The model under review builds one solid part; all positions refer to its coordinate system, in mm. Face numbers are marked on the shaded views. A direction names the side the tool comes from. Coordinates: 2 decimals unless noted, no trailing zeros. Loops run counter-clockwise (first coordinate to the right, second up) from the corner with the lowest first, then second, coordinate; pieces in that order, holes last. Notation, with made-up numbers: (33.25, 49) - (85.25, 49) arc R18 cw to (85.25, 56) - close; hole circle Ø5 at (51, 79). An arc over 180 degrees is marked (long way). Answer in a Markdown table with one row per item. Add a question column.
(1) Mouldability with a two-part tool opening along X and no side actions: class the marked faces 3, 4, 5 and 6 as +X half, -X half, draft (parallel to the pull), parting line (faces both ways), or undercut.
(2) We need section A-A on z = 11.5. Write out the cut boundary in (x, y).
(3) For line 1 along X through (y, z) = (-11.5, 9.75); line 2 along X through (y, z) = (-16, 0.5); line 3 along Z through (x, y) = (2, -21.5), list the stretches that pass through material, from the lowest coordinate up.
(4) We need section D-D on y = -2.5. Write out the cut boundary in (x, z), plus the area to 3 significant figures.
(5) Machinability: for the marked faces 1 and 2, which of the approach directions +Z, -Z, +X, -X, +Y, -Y give a long, thin tool a straight path to every point of the face, cutting with its end or side? Answer none if there is none.
(6) For P1, Ø0.6, axis at x = 0.5, y = -20, coming from the +Z side; P2, Ø2, axis at x = 0, y = -12, coming from the +Z side; P3, Ø1.6, axis at x = -0.5, z = 12.5, coming from the -Y side; P4, Ø2, axis at y = -4, z = -10.5, coming from the +X side, all flat-tipped, find the tip position at first contact; note any pin that passes through.
(7) We need section C-C on y = -23. Write out the cut boundary in (x, z), plus the area to 3 significant figures.
from build123d import *

# Parameters (mm, degrees)
F0_W     = 14
F0_H     = 5
F1_DEPTH = 2
F2_W     = 13
F2_H     = 5
F3_DEPTH = 31
F4_W     = 2
F4_H     = 1.2
F5_DEPTH = 2


with BuildPart() as f1:
    # F0 (on Front) → F1 (new body)
    with BuildSketch(Plane.XZ):
        Polygon((2.468578, 14), (-2.468578, 14), (-7.107986, 12.311393), (-10.890067, 9.137851), (-13.358645, 4.862149), (-14.215973, 0), (-13.358645, -4.862149), (-10.890067, -9.137851), (-7.107986, -12.311393), (-2.468578, -14), (2.468578, -14), (7.107986, -12.311393), (10.890067, -9.137851), (13.358645, -4.862149), (14.215973, 0), (13.358645, 4.862149), (10.890067, 9.137851), (7.107986, 12.311393), align=None)
        with BuildLine():
            ThreePointArc((1, 8.944272), (6.708204, 6), (9, 0))
            ThreePointArc((9, 0), (-6, -6.708204), (-1, 8.944272))
            Line((-1, 8.944272), (-1, 10.944272))
            Line((-1, 10.944272), (1, 10.944272))
            Line((1, 10.944272), (1, 8.944272))
        make_face(mode=Mode.SUBTRACT)
        with BuildLine():
            ThreePointArc((-1, 8.944272), (0, 9), (1, 8.944272))
            Line((1, 8.944272), (1, 10.944272))
            Line((1, 10.944272), (-1, 10.944272))
            Line((-1, 10.944272), (-1, 8.944272))
        make_face()
        with BuildLine():
            ThreePointArc((-1, 8.944272), (-6, -6.708204), (9, 0))
            ThreePointArc((9, 0), (6.708204, 6), (1, 8.944272))
            ThreePointArc((1, 8.944272), (0, 9), (-1, 8.944272))
        make_face()
        Rectangle(F0_W, F0_H, mode=Mode.SUBTRACT)
        Rectangle(F0_W, F0_H)
    extrude(amount=F1_DEPTH)

    # F2 (on Front) → F3 (join)
    with BuildSketch(Plane.XZ):
        with BuildLine():
            Line((-1, 10.944272), (-1, 8.944272))
            ThreePointArc((-1, 8.944272), (0, -9), (1, 8.944272))
            Line((1, 8.944272), (1, 10.944272))
            Line((1, 10.944272), (-1, 10.944272))
        make_face()
        Rectangle(F2_W, F2_H, mode=Mode.SUBTRACT)
    extrude(amount=F3_DEPTH)

    # F4 (on face) → F5 (join)
    with BuildSketch(Plane.XY.offset(10.944272)):
        Polygon((1, -4), (1, -2), (-1, -2), (-1, -4), (-1, -5.2), (1, -5.2), align=None)
        Polygon((1, -9.2), (1, -8), (-1, -8), (-1, -9.2), (-1, -10.4), (1, -10.4), align=None)
        with Locations((0, -13.8)):
            Rectangle(F4_W, F4_H)
        with Locations((0, -15)):
            Rectangle(F4_W, F4_H)
        with Locations((0, -19)):
            Rectangle(F4_W, F4_H)
        with Locations((0, -20.2)):
            Rectangle(F4_W, F4_H)
        with Locations((0, -24.2)):
            Rectangle(F4_W, F4_H)
        with Locations((0, -25.4)):
            Rectangle(F4_W, F4_H)
        with Locations((0, -29.4)):
            Rectangle(F4_W, F4_H)
    extrude(amount=F5_DEPTH)


solid = f1.part
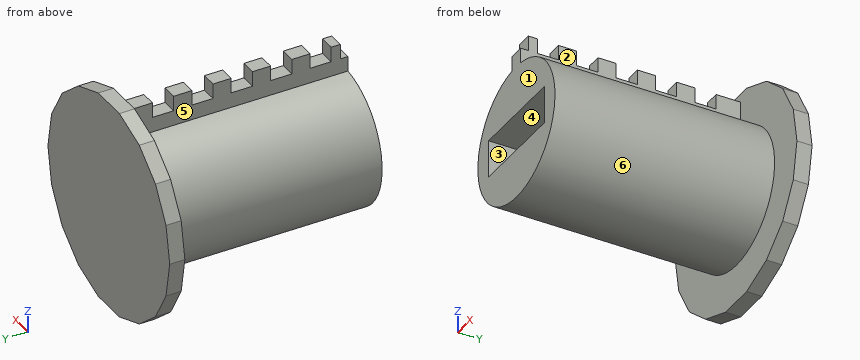
Outcome:
| question | item | result |
|---|---|---|
| 1 | face 3 | undercut |
| 1 | face 4 | undercut |
| 1 | face 5 | -X half |
| 1 | face 6 | parting line |
| 2 | outline | (-8.07, -2) - (-1, -2) - (-1, -5.2) - (1, -5.2) - (1, -2) - (8.07, -2) - (8.07, 0) - (-8.07, 0) - close; (-1, -30) - (1, -30) - (1, -28.8) - (-1, -28.8) - close; (-1, -26) - (1, -26) - (1, -23.6) - (-1, -23.6) - close; (-1, -20.8) - (1, -20.8) - (1, -18.4) - (-1, -18.4) - close; (-1, -15.6) - (1, -15.6) - (1, -13.2) - (-1, -13.2) - close; (-1, -10.4) - (1, -10.4) - (1, -8) - (-1, -8) - close |
| 3 | line 1 | -1 to 1 |
| 3 | line 2 | -8.99 to -6.5, 6.5 to 8.99 |
| 3 | line 3 | -8.77 to -2.5, 2.5 to 8.77 |
| 4 | outline | (-1, 8.94) arc R9 ccw (long way) to (1, 8.94) - (1, 12.94) - (-1, 12.94) - close; hole (-6.5, -2.5) - (6.5, -2.5) - (6.5, 2.5) - (-6.5, 2.5) - close |
| 4 | area | 197 mm² |
| 5 | face 1 | +Z, -Z, +X, -X, -Y |
| 5 | face 2 | +Z, +X, -Y |
| 6 | P1 | z = 12.94 |
| 6 | P2 | z = 10.94 |
| 6 | P3 | y = -30 |
| 6 | P4 | through |
| 7 | outline | (-1, 8.94) arc R9 ccw (long way) to (1, 8.94) - (1, 10.94) - (-1, 10.94) - close; hole (-6.5, -2.5) - (6.5, -2.5) - (6.5, 2.5) - (-6.5, 2.5) - close |
| 7 | area | 193 mm² |
